The model under review builds one solid part; all positions refer to its coordinate system, in mm. Face numbers are marked on the shaded views. A direction names the side the tool comes from. Give positions to 0.01 mm unless a question says otherwise; leave off trailing zeros. Loops run counter-clockwise (first coordinate to the right, second up) from the corner with the lowest first, then second, coordinate; pieces in that order, holes last. Notation, with made-up numbers: M 54.25,89 L 65.25,89 A18 ccw 65.25,118 Z; hole C -26,74 d10. An arc over 180 degrees is marked long. One line per item, written item: value. Start each with the question number.
Q1. For pin 1 (2.5 mm diameter, centred on x = 3.81, z = 6.35, fed in from -Y); pin 2 (6 mm diameter, centred on y = 53.5, z = 10.5, fed in from -X); pin 3 (2 mm diameter, centred on y = 23, z = 4.5, fed in from +X), all flat-tipped, find the tip position at first contact; note any pin that passes through.
Q2. To check wall thickness, follow line 1 along X through (y, z) = (7.5, 6.35); line 2 along Y through (x, z) = (2, 11); line 3 along Z through (x, y) = (39, 8). State the ranges of each line that lie inside material, in increasing order. Write a range as from..to.
Q3. For the marked faces 1, 2 and 3, list the 3-axis set-ups (+Z, -Z, +X, -X, +Y, -Y) from which the entire face can be reached by the end or side of a thin tool; tool diameter is ignored.
Q4. We need section B-B on x = 39.37. Write out the cut boundary in (y, z).
Q5. We need section C-C on y = 76. Write out the cut boundary in (x, z), plus the area to 3 significant figures.
Q6. Mouldability with a two-part tool opening along Y and no side actions: class the marked faces 4, 5, 6 and 7 as released by +Y, released by -Y, zero draft, split by the parting line, or undercut.
Q7. We need section A-A on z = 6.35. Write out the cut boundary in (x, y).
Q8. We need section D-D on z = 10. Write out the cut boundary in (x, y).
```python
from build123d import *

# Parameters (mm, degrees)
BOSS_EXTRUDE1_DEPTH = 12.7
CUT_EXTRUDE1_REACH  = 96.929
SKETCH2_R           = 1.651


with BuildPart() as part:
    # Sketch1 → Boss-Extrude1 (new body)
    with BuildSketch(Plane.XY):
        with BuildLine():
            Line((0, 0), (43.18, 0))
            Line((43.18, 0), (43.18, 10.990448657))
            Line((43.18, 10.990448657), (34.76788921, 10.990448657))
            Line((34.76788921, 10.990448657), (34.76788921, 61.790448657))
            Line((34.76788921, 61.790448657), (43.18, 61.790448657))
            Line((43.18, 61.790448657), (43.18, 83.580070377))
            Line((43.18, 83.580070377), (33.063937135, 83.580070377))
            ThreePointArc((33.063937135, 83.580070377), (21.59, 68.690045143), (10.116062865, 83.580070377))
            Line((10.116062865, 83.580070377), (0, 83.580070377))
            Line((0, 83.580070377), (0, 61.790448657))
            Line((0, 61.790448657), (8.41211079, 61.790448657))
            Line((8.41211079, 61.790448657), (8.41211079, 12.217122928))
            Line((8.41211079, 12.217122928), (0, 12.217122928))
            Line((0, 12.217122928), (0, 0))
        make_face()
    extrude(amount=BOSS_EXTRUDE1_DEPTH)

    # Sketch2 → Cut-Extrude1 (cut, up to next)
    with BuildSketch(Plane.XZ, mode=Mode.PRIVATE) as cut_extrude1_sk1:
        with Locations(Location((3.81, 6.35, 0), (0, 0, 270))):
            Circle(SKETCH2_R)
    cut_extrude1_tool1 = extrude(cut_extrude1_sk1.sketch, amount=-CUT_EXTRUDE1_REACH, mode=Mode.PRIVATE) & part.part
    # Sketch2 → Cut-Extrude1 (cut, up to next)
    with BuildSketch(Plane.XZ, mode=Mode.PRIVATE) as cut_extrude1_sk2:
        with Locations(Location((39.37, 6.35, 0), (0, 0, 270))):
            Circle(SKETCH2_R)
    cut_extrude1_tool2 = extrude(cut_extrude1_sk2.sketch, amount=-CUT_EXTRUDE1_REACH, mode=Mode.PRIVATE) & part.part
    add(cut_extrude1_tool1.solids().sort_by_distance((3.81, 0, 6.35))[0], mode=Mode.SUBTRACT)
    add(cut_extrude1_tool2.solids().sort_by_distance((39.37, 0, 6.35))[0], mode=Mode.SUBTRACT)


solid = part.part
```
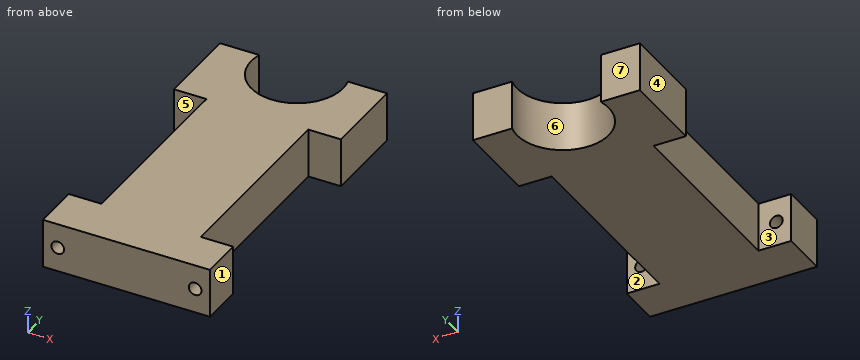
Solved:
1. pin 1: y = 61.79
1. pin 2: x = 8.41
1. pin 3: x = 34.77
2. line 1: 0..2.16, 5.46..37.72, 41.02..43.18
2. line 2: 0..12.22, 61.79..83.58
2. line 3: 0..4.74, 7.96..12.7
3. face 1: +Z, -Z, +X, +Y, -Y
3. face 2: +Z, -Z, +X
3. face 3: +Z, -Z, -X
4. outline: M 0,0 L 10.99,0 L 10.99,4.7 L 0,4.7 Z; M 0,8 L 10.99,8 L 10.99,12.7 L 0,12.7 Z; M 61.79,0 L 83.58,0 L 83.58,12.7 L 61.79,12.7 Z
5. outline: M 0,0 L 10.63,0 L 10.63,12.7 L 0,12.7 Z; M 32.55,0 L 43.18,0 L 43.18,12.7 L 32.55,12.7 Z
5. area: 270 mm2
6. face 4: zero draft
6. face 5: undercut
6. face 6: undercut
6. face 7: released by +Y
7. outline: M 0,0 L 2.16,0 L 2.16,12.22 L 0,12.22 Z; M 0,61.79 L 8.41,61.79 L 8.41,12.22 L 5.46,12.22 L 5.46,0 L 37.72,0 L 37.72,10.99 L 34.77,10.99 L 34.77,61.79 L 43.18,61.79 L 43.18,83.58 L 33.06,83.58 A11.87 cw long 10.12,83.58 L 0,83.58 Z; M 41.02,0 L 43.18,0 L 43.18,10.99 L 41.02,10.99 Z
8. outline: M 0,0 L 43.18,0 L 43.18,10.99 L 34.77,10.99 L 34.77,61.79 L 43.18,61.79 L 43.18,83.58 L 33.06,83.58 A11.87 cw long 10.12,83.58 L 0,83.58 L 0,61.79 L 8.41,61.79 L 8.41,12.22 L 0,12.22 Z
